```python
from build123d import *

# Parameters (mm, degrees)
BOSS_EXTRUDE1_START     = -3
BOSS_EXTRUDE1_OUTLINE_R = 1.25
BOSS_EXTRUDE1_DEPTH     = 3
SKETCH6_W               = 3
SKETCH6_H               = 29.12999922
BOSS_EXTRUDE3_DEPTH     = 11.68
SKETCH9_R               = 1.75
CUT_EXTRUDE2_DEPTH      = 5
BOSS_EXTRUDE4_DEPTH     = 15
SKETCH11_W              = 8
SKETCH11_H              = 3
CUT_EXTRUDE4_DEPTH      = 10


# Read off the part's stored shape, not the designer's step: Boss-Extrude1
with BuildPart() as part:
    # Boss-Extrude1 outline → Boss-Extrude1 (new body)
    with BuildSketch(Plane(origin=(0, 0, 0), x_dir=(1, 0, 0), z_dir=(0, 1, 0)).offset(BOSS_EXTRUDE1_START)):
        with BuildLine():
            Line((21.162477615, -57.094438481), (21.162544036, -28.414715022))
            Line((21.162544036, -28.414715022), (9.924191255, 3.512841719))
            ThreePointArc((9.924191255, 3.512841719), (0, 10.527565199), (-9.924191255, 3.512841719))
            Line((-9.924191255, 3.512841719), (-22.339897891, -28.212185032))
            Line((-22.339897891, -28.212185032), (-22.388445596, -57.094438481))
            Line((-22.388445596, -57.094438481), (21.162477615, -57.094438481))
        make_face()
        with Locations((-3.499861001, -7.487216855)):
            Circle(BOSS_EXTRUDE1_OUTLINE_R, mode=Mode.SUBTRACT)
        with Locations((-7.42819985, -3.486548919)):
            Circle(BOSS_EXTRUDE1_OUTLINE_R, mode=Mode.SUBTRACT)
        with Locations((-7.499989222, 0.012714758)):
            Circle(BOSS_EXTRUDE1_OUTLINE_R, mode=Mode.SUBTRACT)
        with Locations((-7.500049059, 3.512714758)):
            Circle(BOSS_EXTRUDE1_OUTLINE_R, mode=Mode.SUBTRACT)
        with Locations((-3.500117445, 7.512783142)):
            Circle(BOSS_EXTRUDE1_OUTLINE_R, mode=Mode.SUBTRACT)
        with Locations((0.000138999, -7.487157018)):
            Circle(BOSS_EXTRUDE1_OUTLINE_R, mode=Mode.SUBTRACT)
        with Locations((3.499402676, -7.415367646)):
            Circle(BOSS_EXTRUDE1_OUTLINE_R, mode=Mode.SUBTRACT)
        with Locations((7.500070612, -3.487028797)):
            Circle(BOSS_EXTRUDE1_OUTLINE_R, mode=Mode.SUBTRACT)
        with Locations((7.500010775, 0.012971203)):
            Circle(BOSS_EXTRUDE1_OUTLINE_R, mode=Mode.SUBTRACT)
        with Locations((-0.000117446, 7.512842979)):
            Circle(BOSS_EXTRUDE1_OUTLINE_R, mode=Mode.SUBTRACT)
        with Locations((3.499882554, 7.512902816)):
            Circle(BOSS_EXTRUDE1_OUTLINE_R, mode=Mode.SUBTRACT)
        with Locations((7.500070612, 3.512971202)):
            Circle(BOSS_EXTRUDE1_OUTLINE_R, mode=Mode.SUBTRACT)
    extrude(amount=BOSS_EXTRUDE1_DEPTH)

    # Sketch6 → Boss-Extrude3 (add)
    with BuildSketch(Plane.XZ.offset(3)):
        with Locations((-5, 42.529438871)):
            Rectangle(SKETCH6_W, SKETCH6_H)
    extrude(amount=-BOSS_EXTRUDE3_DEPTH)

    # Sketch9 → Cut-Extrude2 (cut)
    with BuildSketch(Plane(origin=(-3.5, 0, 0), x_dir=(0, 0, -1), z_dir=(1, 0, 0))):
        with Locations((-37.369439261, 3.88)):
            Circle(SKETCH9_R)
        with Locations((-47.719439261, 3.88)):
            Circle(SKETCH9_R)
    extrude(amount=-CUT_EXTRUDE2_DEPTH, mode=Mode.SUBTRACT)

    # Sketch10 → Boss-Extrude4 (add)
    with BuildSketch(Plane.XY.offset(57.094438481)):
        Polygon((-22.388445596, 0), (-6.5, 0), (-3.5, 0), (21.162477615, 0), (21.162477615, -3), (-22.388445596, -3), align=None)
    extrude(amount=BOSS_EXTRUDE4_DEPTH)

    # Sketch11 → Cut-Extrude4 (cut)
    with BuildSketch(Plane(origin=(0, 0, 0), x_dir=(1, 0, 0), z_dir=(0, 1, 0))):
        with Locations((-6, -23.5)):
            Rectangle(SKETCH11_W, SKETCH11_H)
    extrude(amount=-CUT_EXTRUDE4_DEPTH, mode=Mode.SUBTRACT)


solid = part.part
```
The listing builds one solid part. Answer for the finished solid, in the listing's coordinates (mm). A direction names the side the tool comes from. Coordinates: 2 decimals unless noted, no trailing zeros. Write each loop counter-clockwise with the first axis right and the second up, starting at its lowest first coordinate (ties: lowest second). Pieces come first, ordered by that corner, then holes. Notation, with made-up numbers: (-28, 68) - (-21, 68) arc R24 ccw to (-21, 90) - close; hole circle Ø11 at (-17.5, 62.5). An arc over 180 degrees is marked (long way). Return JSON: item names as keys, results as strings. Group by question number.
1. Determine the mould class of faces 1 (the flat face through (-3.5, 4, 42)), 2 (the cylindrical face through (0.181, -1.521, -10.526)), 3 (the flat face through (-6, -1, 25)) for opening direction Z: released by +Z, released by -Z, zero draft, split by the parting line, or undercut.
2. A cutting plane is placed at B-B, the plane z = 66. Determine the outline of the cut face in (x, y), plus the area to 3 significant figures.
3. Given pin 1 (6 mm diameter, centred on x = -14.5, z = 34.5, fed in from +Y); pin 2 (0.9 mm diameter, centred on x = -5, y = 6, fed in from +Z); pin 3 (1.5 mm diameter, centred on x = -5, y = 6, fed in from -Z); pin 4 (2 mm diameter, centred on y = 3.88, z = 47.72, fed in from +X), each flat-ended and moving along its own axis, determine where each tip first touches the part or whether it passes through.
4. Which of the six approach directions +Z, -Z, +X, -X, +Y, -Y give full straight-line access (tool end or side, diameter ignored) to faces 4 (the flat face through (-2, -1, 24)), 5 (the flat face through (0, -3, 39))?
5. Straight lines are drawn through the part: L1, parallel to X at y = -0.5, z = -4.5; L2, parallel to Z at x = 2.5, y = -1; L3, parallel to Y at x = -8, z = 32. For each, find the intervals that lie inside material, in ascending order.
6. A cutting plane is placed at A-A, the plane y = 3.88. Determine the outline of the cut face in (x, z), plus the area to 3 significant figures.
7. A cutting plane is placed at C-C, the plane x = -17. Determine the outline of the cut face in (y, z), plus the area to 3 significant figures.
Ans:
{
 "1": {"face 1": "zero draft", "face 2": "released by -Z", "face 3": "undercut"},
 "2": {"outline": "(-22.39, -3) - (21.16, -3) - (21.16, 0) - (-22.39, 0) - close", "area": "131 mm²"},
 "3": {"pin 1": "y = 0", "pin 2": "z = 57.09", "pin 3": "z = 27.96", "pin 4": "through"},
 "4": {"face 4": "+Y, -Y", "face 5": "+Z, -Z, +X, -X, -Y"},
 "5": {"L1": "-9.52 to -8.27, -6.73 to 6.73, 8.27 to 9.52", "L2": "-10.23 to -8.26, -6.76 to 6.66, 8.17 to 72.09", "L3": "-3 to 0"},
 "6": {"outline": "(-6.5, 27.96) - (-3.5, 27.96) - (-3.5, 35.62) - (-6.5, 35.62) - close; (-6.5, 39.12) - (-3.5, 39.12) - (-3.5, 45.97) - (-6.5, 45.97) - close; (-6.5, 49.47) - (-3.5, 49.47) - (-3.5, 57.09) - (-6.5, 57.09) - close", "area": "66.4 mm²"},
 "7": {"outline": "(-3, 14.57) - (0, 14.57) - (0, 72.09) - (-3, 72.09) - close", "area": "173 mm²"}
}
